Can you work these out from the model? Positions are in its coordinate system, mm. A direction names the side the tool comes from. Coordinates: 2 decimals unless noted, no trailing zeros. Loops run counter-clockwise (first coordinate to the right, second up) from the corner with the lowest first, then second, coordinate; pieces in that order, holes last.
```python
from build123d import *

# Parameters (mm, degrees)
F2_DEPTH        = 210
F4_W            = 185.4063174448
F4_H            = 139
F5_DEPTH        = 6
F4_W_2          = 191.4063174448
F4_H_2          = 145
F6_DEPTH        = 2
F7_W            = 45.5
F7_H            = 140.02
F7_W_2          = 39.5
F7_H_2          = 134.02
F8_DEPTH        = 12
F9_DEPTH        = 9
F10_DEPTH       = 3
F3_R            = 7.5
F11_DEPTH       = 16
F12_D           = 4.5
F12_DEPTH       = 40
F12_CBORE_D     = 8
F12_CBORE_DEPTH = 4.5
F12_TIP         = 1.3519363928


with BuildPart() as f2:
    # F1 (on Front) → F2 (new body)
    with BuildSketch(Plane.XZ):
        Polygon((50.8599747535, 131), (-6, 131), (-6, -6), (279.3492325705, -6), (242.2383099785, 74.989177444), align=None)
        Polygon((240.0814283237, 72.494588722), (274.6746162852, -3), (-3, -3), (-3, 128), (50.4299873767, 128), align=None, mode=Mode.SUBTRACT)
        Polygon((-3, -3), (274.6746162852, -3), (240.0814283237, 72.494588722), (50.4299873767, 128), (-3, 128), align=None)
        Polygon((270, 0), (0, 0), (0, 125), (50, 125), (237.9245466688, 70), align=None, mode=Mode.SUBTRACT)
    extrude(amount=-F2_DEPTH)

    # F4 (on face) → F5 (cut, through all)
    with BuildSketch(Plane(origin=(39.3276682275, 0, 134.3751676945), x_dir=(0.9597405823, 0, -0.280887904), z_dir=(0.280887904, 0, 0.9597405823))):
        with Locations((112.7192250827, 77.5)):
            Rectangle(F4_W, F4_H)
    extrude(amount=-F5_DEPTH, mode=Mode.SUBTRACT)

    # F4 (on face) → F6 (cut)
    with BuildSketch(Plane(origin=(39.3276682275, 0, 134.3751676945), x_dir=(0.9597405823, 0, -0.280887904), z_dir=(0.280887904, 0, 0.9597405823))):
        with Locations((112.7192250827, 77.5)):
            Rectangle(F4_W_2, F4_H_2)
        with Locations((112.7192250827, 77.5)):
            Rectangle(F4_W, F4_H, mode=Mode.SUBTRACT)
    extrude(amount=-F6_DEPTH, mode=Mode.SUBTRACT)

    # F7 (on face) → F8 (join)
    with BuildSketch(Plane.XY.offset(131)):
        with Locations((22.4299873767, 75.6899873767)):
            Rectangle(F7_W, F7_H)
        with Locations((22.4299873767, 75.6899873767)):
            Rectangle(F7_W_2, F7_H_2, mode=Mode.SUBTRACT)
        with Locations((22.4299873767, 75.6899873767)):
            Rectangle(F7_W_2, F7_H_2)
    extrude(amount=-F8_DEPTH)

    # F7 (on face) → F9 (cut)
    with BuildSketch(Plane.XY.offset(131)):
        with Locations((22.4299873767, 75.6899873767)):
            Rectangle(F7_W_2, F7_H_2)
    extrude(amount=-F9_DEPTH, mode=Mode.SUBTRACT)

    # F1 (on Front) → F10 (cut)
    with BuildSketch(Plane.XZ):
        Polygon((-3, -3), (274.6746162852, -3), (240.0814283237, 72.494588722), (50.4299873767, 128), (-3, 128), align=None)
        Polygon((270, 0), (0, 0), (0, 125), (50, 125), (237.9245466688, 70), align=None, mode=Mode.SUBTRACT)
    extrude(amount=-F10_DEPTH, mode=Mode.SUBTRACT)

    # F3 (on face) → F11 (join)
    with BuildSketch(Plane(origin=(0, 0, -6), x_dir=(1, 0, 0), z_dir=(0, 0, -1))):
        with Locations((192.9705612659, -177.0294387341)):
            Circle(F3_R)
        with Locations((192.9705612659, -127.0294387341)):
            Circle(F3_R)
        with Locations((42.9705612659, -177.0294387341)):
            Circle(F3_R)
        with Locations((42.9705612659, -127.0294387341)):
            Circle(F3_R)
    extrude(amount=-F11_DEPTH)

    # F12
    with Locations(Plane(origin=(0, 0, -6), x_dir=(1, 0, 0), z_dir=(0, 0, -1))):
        with Locations((192.9705612659, -127.0294387341), (192.9705612659, -177.0294387341), (42.9705612659, -177.0294387341), (42.9705612659, -127.0294387341)):
            CounterBoreHole(F12_D / 2, F12_CBORE_D / 2, F12_CBORE_DEPTH, depth=F12_DEPTH)
            with Locations((0, 0, -(F12_DEPTH + F12_TIP / 2))):  # 118° drill point
                Cone(0, F12_D / 2, F12_TIP, mode=Mode.SUBTRACT)


solid = f2.part
```
Item 1: I need wall thicknesses on line 1 along Z through (x, y) = (8, 160); line 2 along Z through (x, y) = (7, 92); line 3 along X through (y, z) = (76.5, 83.5). Which ranges of each line are inside material? Lowest first, please.
Results are:
line 1: z = -6 to 0, 125 to 131
line 2: z = -6 to 0, 119 to 122
line 3: x = -6 to 0
Item 2: On a 3-axis mill with a long thin cutter (end or side, diameter ignored), from which of +Z, -Z, +X, -X, +Y, -Y can I reach the whole of each face in a straight line? I mean faces 1 (the face through (197.003, 170.705, 4.93)), 2 (the face through (45, 129, -1.5)), 3 (the face through (135.2, 3, -0.3)), 4 (the face through (22, 145.7, 122)), 5 (the face through (42.18, 75, 127)). Say none if no direction works.
Results are:
face 1: none
face 2: -Z
face 3: -Y
face 4: +Y
face 5: +Z
Item 3: I'm going to push flat-ended pins straight in: P1, Ø7, axis at x = 192.97, y = 127.03, coming from the +Z side; P2, Ø8, axis at x = 166, y = 48, coming from the +Z side; P3, Ø6, axis at x = 42.97, y = 177.03, coming from the -Z side. Where does each tip first touch, or does it pass through?
Results are:
P1: stops at z = 10
P2: stops at z = 0
P3: stops at z = -1.5
Item 4: Suppose I cut it at A-A, the plane y = 193. Please give me the cut outline in (x, z).
Results are:
outline: (-6, -6) - (279.35, -6) - (242.24, 74.99) - (50.86, 131) - (-6, 131) - close; hole (0, 0) - (270, 0) - (237.92, 70) - (50, 125) - (0, 125) - close
Item 5: Suppose I cut it at B-B, the plane z = 96.5. Please give me the cut outline in (x, y), plus the area to 3 significant figures.
Results are:
outline: (-6, 0) - (-3, 0) - (-3, 3) - (0, 3) - (0, 210) - (-6, 210) - close; (147.38, 3) - (158.06, 3) - (158.06, 0) - (168.74, 0) - (168.74, 5) - (161.62, 5) - (161.62, 8) - (147.38, 8) - close; (147.38, 147) - (161.62, 147) - (161.62, 150) - (168.74, 150) - (168.74, 210) - (147.38, 210) - close
area: 2,690 mm2
Item 6: Suppose I cut it at C-C, the plane x = 103. Please give me the cut outline in (y, z), plus the area to 3 significant figures.
Results are:
outline: (0, -6) - (210, -6) - (210, 0) - (3, 0) - (3, -3) - (0, -3) - close; (0, 112.61) - (3, 112.61) - (3, 109.49) - (8, 109.49) - (8, 113.66) - (5, 113.66) - (5, 115.74) - (0, 115.74) - close; (147, 109.49) - (210, 109.49) - (210, 115.74) - (150, 115.74) - (150, 113.66) - (147, 113.66) - close
area: 1,670 mm2
Item 7: We'd pull the mould along X, two halves only. Please class faces 6 (the face through (22, 153, 131)), 7 (the face through (45, 125, 10)): +X half, -X half, draft (parallel to the pull), parting line (faces both ways), or undercut.
Results are:
face 6: draft
face 7: undercut
Item 8: Suppose I cut it at D-D, the plane z = 17.5. Please give me the cut outline in (x, y), plus the area to 3 significant figures.
Results are:
outline: (-6, 0) - (-3, 0) - (-3, 3) - (0, 3) - (0, 210) - (-6, 210) - close; (261.98, 3) - (265.28, 3) - (265.28, 0) - (268.58, 0) - (268.58, 210) - (261.98, 210) - close
area: 2,630 mm2
